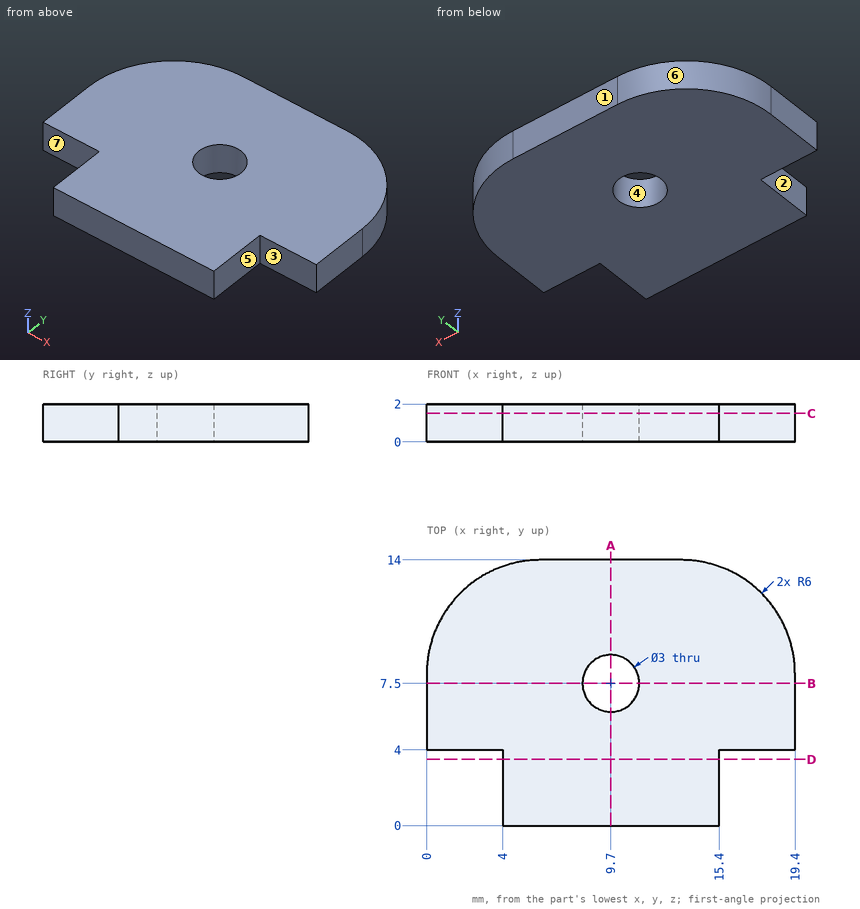
Answer from the drawing. Dimensions are ordinates in mm from the lowest x, y and z of the part. A direction names the side the tool comes from. Round coordinates to 2 decimals unless told otherwise and drop trailing zeros. Write each loop counter-clockwise with the first axis right and the second up, starting at its lowest first coordinate (ties: lowest second). Pieces come first, ordered by that corner, then holes. Notation, with made-up numbers: (-14, 17) - (12, 17) arc R16 cw to (12, 21) - close; hole circle Ø6 at (25, 69). An arc over 180 degrees is marked (long way). Use a Markdown table: item, result.
(1) Straight lines are drawn through the part: line 1 along Y through (x, z) = (9.7, 0.6); line 2 along X through (y, z) = (3.25, 0.1); line 3 along X through (y, z) = (7, 0.2). For each, find the intervals that lie inside material, in ascending order. Write a range as [from, to].
Reported:
| item | result |
|---|---|
| line 1 | [0, 6], [9, 14] |
| line 2 | [4, 15.4] |
| line 3 | [0, 8.29], [11.11, 19.4] |
(2) Each of these flat-tipped pins is pushed along its axis until it touches: pin 1 Ø0.6 at (x, z) = (18, 1) entering from -Y; pin 2 Ø0.6 at (y, z) = (2, 0.5) entering from +X. Where does it stop, or does it pass through?
Reported:
| item | result |
|---|---|
| pin 1 | y = 4 |
| pin 2 | x = 15.4 |
(3) The part is cut by section B-B (y = 7.5). Write down the section's boundary in (x, z).
Reported:
| item | result |
|---|---|
| outline | (0, 0) - (8.2, 0) - (8.2, 2) - (0, 2) - close; (11.2, 0) - (19.4, 0) - (19.4, 2) - (11.2, 2) - close |
(4) The part is cut by section D-D (y = 3.5). Write down the section's boundary in (x, z), then the cut area to 3 significant figures.
Reported:
| item | result |
|---|---|
| outline | (4, 0) - (15.4, 0) - (15.4, 2) - (4, 2) - close |
| area | 22.8 mm2 |
(5) Which of the six approach directions +Z, -Z, +X, -X, +Y, -Y give full straight-line access (tool end or side, diameter ignored) to the marked faces 1, 2 and 3?
Reported:
| item | result |
|---|---|
| face 1 | +Z, -Z, +X, -X, +Y |
| face 2 | +Z, -Z, -X, -Y |
| face 3 | +Z, -Z, +X, -Y |
(6) The part is cut by section C-C (z = 1.5). Write down the section's boundary in (x, y).
Reported:
| item | result |
|---|---|
| outline | (0, 4) - (4, 4) - (4, 0) - (15.4, 0) - (15.4, 4) - (19.4, 4) - (19.4, 8) arc R6 ccw to (13.4, 14) - (6, 14) arc R6 ccw to (0, 8) - close; hole circle Ø3 at (9.7, 7.5) |
(7) The mould has two halves that part along X. Classify the marked faces 4, 5, 6 and 7: released by +X, released by -X, zero draft, split by the parting line, or undercut.
Reported:
| item | result |
|---|---|
| face 4 | undercut |
| face 5 | released by +X |
| face 6 | released by -X |
| face 7 | zero draft |
(8) The part is cut by section A-A (x = 9.7). Write down the section's boundary in (y, z).
Reported:
| item | result |
|---|---|
| outline | (0, 0) - (6, 0) - (6, 2) - (0, 2) - close; (9, 0) - (14, 0) - (14, 2) - (9, 2) - close |
